The listing builds one solid part. Answer for the finished solid, in the listing's coordinates (mm). A direction names the side the tool comes from. Give positions to 0.01 mm unless a question says otherwise; leave off trailing zeros. Loops run counter-clockwise (first coordinate to the right, second up) from the corner with the lowest first, then second, coordinate; pieces in that order, holes last. Notation, with made-up numbers: (48.25, -31) - (75.25, -31) arc R33 cw to (75.25, 8) - close; hole circle Ø8 at (-33.75, -2.5). An arc over 180 degrees is marked (long way). One line per item, written item: value. Start each with the question number.
from build123d import *

# Parameters (mm, degrees)
SKETCH_1_W          = 56
SKETCH_1_H          = 80
SKETCH_1_W_2        = 3
SKETCH_1_H_2        = 15
SKETCH_1_W_3        = 20
SKETCH_1_H_3        = 3
EXTRUDE_1_DEPTH     = 3
SKETCH_2_W          = 15
SKETCH_2_H          = 3
CUT_EXTRUDE_1_DEPTH = 3
SKETCH_3_W          = 8
SKETCH_3_H          = 80
EXTRUDE_2_DEPTH     = 3
SKETCH_4_W          = 9
SKETCH_4_H          = 3
CUT_EXTRUDE_2_DEPTH = 3
CHAMFER_1_SIZE      = 15


with BuildPart() as part:
    # 草图1 → 凸台-拉伸1 (new body)
    # profile 1 of 2: a face of its own
    with BuildSketch(Plane.XY):
        Rectangle(SKETCH_1_W, SKETCH_1_H)
        with Locations((21.5, 12.5)):
            Rectangle(SKETCH_1_W_2, SKETCH_1_H_2, mode=Mode.SUBTRACT)
        with Locations((21.5, -17.5)):
            Rectangle(SKETCH_1_W_2, SKETCH_1_H_2, mode=Mode.SUBTRACT)
        with Locations((-21.5, -17.5)):
            Rectangle(SKETCH_1_W_2, SKETCH_1_H_2, mode=Mode.SUBTRACT)
        with Locations((-21.5, 12.5)):
            Rectangle(SKETCH_1_W_2, SKETCH_1_H_2, mode=Mode.SUBTRACT)
    # profile 2 of 2: a face of its own
    with BuildSketch(Plane.XY):
        with Locations((0, -41.5)):
            Rectangle(SKETCH_1_W_3, SKETCH_1_H_3)
    extrude(amount=EXTRUDE_1_DEPTH)

    # 草图2 → 切除-拉伸1 (cut)
    with BuildSketch(Plane.XY.offset(3)):
        with Locations((0, -21.5)):
            Rectangle(SKETCH_2_W, SKETCH_2_H)
    extrude(amount=-CUT_EXTRUDE_1_DEPTH, mode=Mode.SUBTRACT)

    # 草图3 → 凸台-拉伸2 (add)
    with BuildSketch(Plane.XY.offset(3)):
        with Locations((-32, 0)):
            Rectangle(SKETCH_3_W, SKETCH_3_H)
    extrude(amount=-EXTRUDE_2_DEPTH)

    # 草图4 → 切除-拉伸2 (cut)
    with BuildSketch(Plane.XY.offset(3)):
        with Locations((-31.5, -21.5)):
            Rectangle(SKETCH_4_W, SKETCH_4_H)
    extrude(amount=-CUT_EXTRUDE_2_DEPTH, mode=Mode.SUBTRACT)

    # 倒角1
    chamfer_1_edges = [part.edges().sort_by_distance(p)[0] for p in [
        (-36, 40, 1.5),
    ]]
    chamfer(chamfer_1_edges, length=CHAMFER_1_SIZE)


solid = part.part
1. A cutting plane is placed at B-B (z = 2.5). Give the number of separate pieces and of enclosed holes in the cut face, plus the area to 3 significant figures.
2. Find the intervals of material crossed by L1, parallel to X at y = 19, z = 1.3; L2, parallel to Y at x = -20.5, z = 1.4; L3, parallel to Y at x = 2, z = 2.95, in increasing order. Write a range as [from, to].
3. For faces 4 (the flat face through (-23, -40, 2)), 5 (the flat face through (-32, -23, 2)), 6 (the flat face through (21, 20, 1)), determine the directions among +Z, -Z, +X, -X, +Y, -Y from which every point of the face is accessible in a straight line to the end or side of a thin tool.
4. A cutting plane is placed at C-C (x = -17). Determine the outline of the cut face in (y, z), plus the area to 3 significant figures.
5. A cutting plane is placed at D-D (y = 34). Determine the outline of the cut face in (x, z), plus the area to 3 significant figures.
6. A cutting plane is placed at A-A (y = 9.5). Determine the outline of the cut face in (x, z).
7. Flat-ended cylindrical pins translate along their axes: pin 1 (0.9 mm diameter, centred on x = -19, z = 1, fed in from -Y); pin 2 (0.9 mm diameter, centred on x = -31.5, z = 2, fed in from +Y); pin 3 (1.5 mm diameter, centred on y = -42, z = 1.5, fed in from -X). Find the tip coordinate at first contact, or state that the pin passes through.
8. Determine the mould class of faces 1 (the flat face through (20, 12, 1)), 2 (the flat face through (-10, -42, 1)), 3 (the flat face through (19, -40, 1)) for opening direction X: released by +X, released by -X, zero draft, split by the parting line, or undercut.
Results below:
1. separate pieces: 1
1. enclosed holes: 5
1. area: 4,820 mm^2
2. L1: x = [-36, -23], [-20, 20], [23, 28]
2. L2: y = [-40, -25], [-10, 5], [20, 40]
2. L3: y = [-43, -23], [-20, 40]
3. face 4: +Z, -Z, -X, -Y
3. face 5: +Z, -Z, -X
3. face 6: +Z, -Z
4. outline: (-40, 0) - (40, 0) - (40, 3) - (-40, 3) - close
4. area: 240 mm^2
5. outline: (-27, 0) - (28, 0) - (28, 3) - (-27, 3) - close
5. area: 165 mm^2
6. outline: (-36, 0) - (-23, 0) - (-23, 3) - (-36, 3) - close; (-20, 0) - (20, 0) - (20, 3) - (-20, 3) - close; (23, 0) - (28, 0) - (28, 3) - (23, 3) - close
7. pin 1: stops at y = -40
7. pin 2: stops at y = 29.95
7. pin 3: stops at x = -10
8. face 1: undercut
8. face 2: released by -X
8. face 3: zero draft
